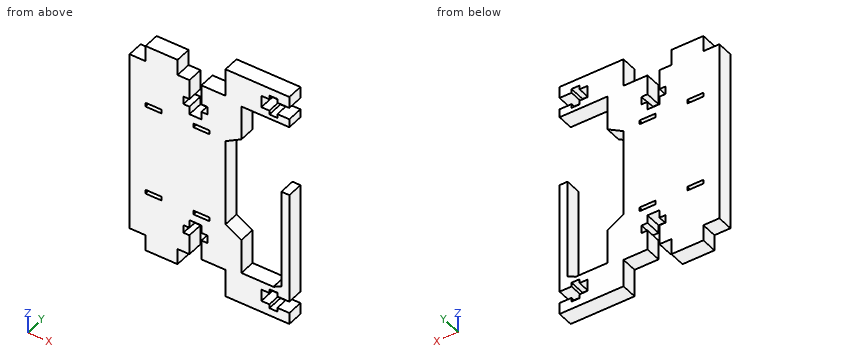
from build123d import *

# Parameters (mm, degrees)
BOSS_EXTRUDE1_DEPTH = 6.35
SKETCH2_W           = 6.35
SKETCH2_H           = 1.5875
CUT_EXTRUDE1_DEPTH  = 6.35
CUT_EXTRUDE2_DEPTH  = 6.35
SKETCH4_W           = 36.519416468
SKETCH4_H           = 95.25
CUT_EXTRUDE5_DEPTH  = 6.35
SKETCH7_W           = 18.153928565
SKETCH7_H           = 28.487742684
CUT_EXTRUDE6_DEPTH  = 6.35


with BuildPart() as part:
    # Sketch1 → Boss-Extrude1 (new body)
    with BuildSketch(Plane(origin=(0, 0, 0), x_dir=(1, 0, 0), z_dir=(0, 1, 0))):
        Polygon((38.1, 65.0875), (66.675, 65.0875), (66.675, -30.1625), (38.1, -30.1625), (38.1, -19.05), (19.05, -19.05), (19.05, -25.4), (6.35, -25.4), (6.35, -19.05), (0, -19.05), (0, 0), (0, 34.925), (0, 53.975), (6.35, 53.975), (6.35, 60.325), (19.05, 60.325), (19.05, 53.975), (38.1, 53.975), align=None)
        Polygon((38.1, 34.925), (44.45, 38.591174209), (44.45, 52.3875), (57.15, 52.3875), (60.325, 50.8), (60.325, -15.875), (57.15, -17.4625), (44.45, -17.4625), (44.45, -3.666174209), (38.1, 0), align=None, mode=Mode.SUBTRACT)
    extrude(amount=BOSS_EXTRUDE1_DEPTH)

    # Sketch2 → Cut-Extrude1 (cut)
    with BuildSketch(Plane(origin=(0, 6.35, 0), x_dir=(1, 0, 0), z_dir=(0, 1, 0))):
        with Locations((9.525, 35.71875)):
            Rectangle(SKETCH2_W, SKETCH2_H)
        with Locations((9.525, -0.79375)):
            Rectangle(SKETCH2_W, SKETCH2_H)
        with Locations((28.575, 35.71875)):
            Rectangle(SKETCH2_W, SKETCH2_H)
        with Locations((28.575, -0.79375)):
            Rectangle(SKETCH2_W, SKETCH2_H)
    extrude(amount=-CUT_EXTRUDE1_DEPTH, mode=Mode.SUBTRACT)

    # Sketch3 → Cut-Extrude2 (cut)
    with BuildSketch(Plane(origin=(0, 6.35, 0), x_dir=(1, 0, 0), z_dir=(0, 1, 0))):
        Polygon((28.549517374, 53.975), (23.787017374, 53.975), (23.787017374, 46.0375), (21.405767374, 46.0375), (21.405767374, 42.8625), (23.787017374, 42.8625), (23.787017374, 39.6875), (28.549517374, 39.6875), (28.549517374, 42.8625), (30.930767374, 42.8625), (30.930767374, 46.0375), (28.549517374, 46.0375), align=None)
        Polygon((66.675, 55.72125), (66.675, 60.48375), (58.7375, 60.48375), (58.7375, 62.07125), (55.5625, 62.07125), (55.5625, 60.48375), (52.3875, 60.48375), (52.3875, 55.72125), (55.5625, 55.72125), (55.5625, 54.13375), (58.7375, 54.13375), (58.7375, 55.72125), align=None)
        Polygon((55.5625, -27.14625), (58.7375, -27.14625), (58.7375, -25.55875), (66.675, -25.55875), (66.675, -20.79625), (58.7375, -20.79625), (58.7375, -19.20875), (55.5625, -19.20875), (55.5625, -20.79625), (52.3875, -20.79625), (52.3875, -25.55875), (55.5625, -25.55875), align=None)
        Polygon((28.549517374, -11.1125), (30.930767374, -11.1125), (30.930767374, -7.9375), (28.549517374, -7.9375), (28.549517374, -4.7625), (23.787017374, -4.7625), (23.787017374, -7.9375), (21.405767374, -7.9375), (21.405767374, -11.1125), (23.787017374, -11.1125), (23.787017374, -19.05), (28.549517374, -19.05), align=None)
    extrude(amount=-CUT_EXTRUDE2_DEPTH, mode=Mode.SUBTRACT)

    # Sketch4 → Cut-Extrude5 (cut)
    with BuildSketch(Plane(origin=(0, 6.35, 0), x_dir=(1, 0, 0), z_dir=(0, 1, 0))):
        with Locations((81.759708234, 17.4625)):
            Rectangle(SKETCH4_W, SKETCH4_H)
    extrude(amount=-CUT_EXTRUDE5_DEPTH, mode=Mode.SUBTRACT)

    # Sketch7 → Cut-Extrude6 (cut)
    with BuildSketch(Plane(origin=(0, 6.35, 0), x_dir=(1, 0, 0), z_dir=(0, 1, 0))):
        with Locations((64.899881691, -3.218628658)):
            Rectangle(SKETCH7_W, SKETCH7_H)
    extrude(amount=-CUT_EXTRUDE6_DEPTH, mode=Mode.SUBTRACT)


solid = part.part
Source: CAD feature listing. Evaluate the final solid. Frame: model axes, mm. Round coordinates to 2 decimals unless told otherwise and drop trailing zeros. Loops run counter-clockwise (first coordinate to the right, second up) from the corner with the lowest first, then second, coordinate; pieces in that order, holes last. Notation, with made-up numbers: (12.5, -20) - (18.5, -20) arc R26 cw to (18.5, 10) - close; hole circle Ø1 at (4.5, 67.25). An arc over 180 degrees is marked (long way). Write item = value, one per line. Start each with the question number.
(1) Section query A-A, the plane x = 46.5. Output: boundary loops of the cut face in (y, z), plus the area to 3 significant figures.
(2) Section query B-B, the plane z = -48.5. Output: boundary loops of the cut face in (x, y) (3 decimals).
(3) Section query C-C, the plane z = 10. Output: boundary loops of the cut face in (x, y).
(4) Pin query (flat end, axial travel): pin 1 (2 mm diameter, centred on x = 11, y = 4.5, fed in from -Z) (3 decimals); pin 2 (0.7 mm diameter, centred on x = 29.5, y = 2.5, fed in from +Z); pin 3 (1 mm diameter, centred on y = 4.5, z = 10, fed in from +X); pin 4 (12 mm diameter, centred on x = 53.5, z = -12.5, fed in from -Y). Return the tip coordinate at first contact, or that it passes through.
(5) Section query D-D, the plane y = 4. State how many separate pieces and enclosed holes the cut face has, plus the area to 3 significant figures.
(6) Ray query, line 1 along X through (y, z) = (2.75, -45) (3 decimals); line 2 along Z through (x, y) = (12, 3.5) (1 decimal); line 3 along X through (y, z) = (4, 20.5). Return the intervals inside material, ascending. Write a range as from..to.
Conclusion:
q1.outline = (0, -65.09) - (6.35, -65.09) - (6.35, -52.39) - (0, -52.39) - close; (0, 17.46) - (6.35, 17.46) - (6.35, 30.16) - (0, 30.16) - close
q1.area = 161 mm2
q2.outline = (0, 0) - (23.787, 0) - (23.787, 6.35) - (0, 6.35) - close; (28.55, 0) - (44.45, 0) - (44.45, 6.35) - (28.55, 6.35) - close; (60.325, 0) - (63.5, 0) - (63.5, 6.35) - (60.325, 6.35) - close
q3.outline = (0, 0) - (21.41, 0) - (21.41, 6.35) - (0, 6.35) - close; (30.93, 0) - (44.45, 0) - (44.45, 6.35) - (30.93, 6.35) - close
q4.pin_1 = -60.325
q4.pin_2 = 19.05
q4.pin_3 = 44.45
q4.pin_4 = through
q5.separate_pieces = 1
q5.enclosed_holes = 4
q5.area = 3,590 mm2
q6.line_1 = 0..21.406, 30.931..44.45, 60.325..63.5
q6.line_2 = -60.3..-36.5, -34.9..0, 1.6..25.4
q6.line_3 = 6.35..19.05, 38.1..55.56, 58.74..63.5
